Part print with two shaded views. Sizes in mm from the minimum x, y, z corner. Give positions to 0.01 mm unless a question says otherwise; leave off trailing zeros. Order: outer loops, then holes, each group sorted by start corner. A loop starts at its lowest first (then second) coordinate and runs counter-clockwise, first axis right, second up. Notation, with made-up numbers: (39, 10.5) -> (70, 10.5) arc R33 ccw to (70, 45.5) -> close; hole circle Ø11 at (63, 8). An arc over 180 degrees is marked (long way). Answer as CSV lines item,"result".
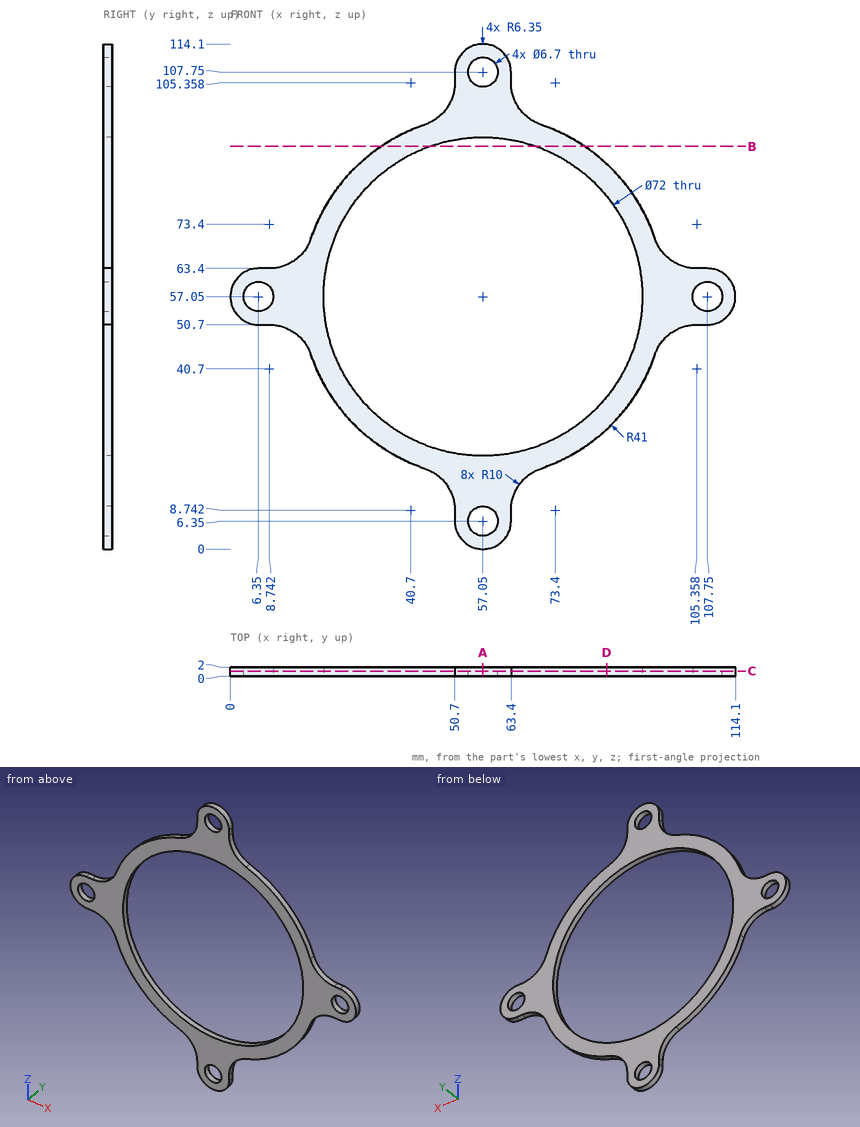
1) Band-saw the part on C-C, the plane y = 1.1. Give the number of separate pieces and of enclosed holes in the cut face, then the cut area to 3 significant figures.
Data:
separate pieces,"1"
enclosed holes,"5"
area,"1,910 mm2"
2) Band-saw the part on A-A, the plane x = 57.05. Write the cut outline in (y, z).
Data:
outline,"(0, 0) -> (2, 0) -> (2, 3) -> (0, 3) -> close; (0, 9.7) -> (2, 9.7) -> (2, 21.05) -> (0, 21.05) -> close; (0, 93.05) -> (2, 93.05) -> (2, 104.4) -> (0, 104.4) -> close; (0, 111.1) -> (2, 111.1) -> (2, 114.1) -> (0, 114.1) -> close"
3) Band-saw the part on D-D, the plane x = 85. Write the cut outline in (y, z).
Data:
outline,"(0, 27.05) -> (2, 27.05) -> (2, 34.36) -> (0, 34.36) -> close; (0, 79.74) -> (2, 79.74) -> (2, 87.05) -> (0, 87.05) -> close"
4) Wall check: line 1 along X through (y, z) = (1.1, 107.75); line 2 along Z through (x, y) = (59, 1.65). Give the ranges that are in metal, low to high. Write a range as [from, to].
Data:
line 1,"x = [50.7, 53.7], [60.4, 63.4]"
line 2,"z = [0.31, 3.63], [9.07, 21.1], [93, 105.03], [110.47, 113.79]"
5) Pin check, flat tips, straight feed: P1, Ø5.5, axis at x = 107.75, z = 57.05, coming from the -Y side (3 decimals); P2, Ø0.6, axis at x = 7, y = 1, coming from the -Z side; P3, Ø1, axis at y = 1, z = 107, coming from the +X side; P4, Ø1, axis at y = 1.5, z = 48, coming from the +X side. Stop position of each tip, or through.
Data:
P1,"passes through"
P2,"stops at z = 50.7"
P3,"stops at x = 63.4"
P4,"stops at x = 99.1"
6) Band-saw the part on B-B, the plane z = 91. Write the cut outline in (x, y) (3 decimals).
Data:
outline,"(34.063, 0) -> (45.075, 0) -> (45.075, 2) -> (34.063, 2) -> close; (69.025, 0) -> (80.037, 0) -> (80.037, 2) -> (69.025, 2) -> close"
